```python
from build123d import *

# Parameters (mm, degrees)
SKETCH1_W           = 76.2
SKETCH1_H           = 101.6
SKETCH1_R           = 2.25
BOSS_EXTRUDE1_DEPTH = 3.175
BOSS_EXTRUDE2_DEPTH = 3.175
SKETCH3_R           = 2.25
CUT_EXTRUDE1_DEPTH  = 10


with BuildPart() as part:
    # Sketch1 → Boss-Extrude1 (new body)
    with BuildSketch(Plane(origin=(0, 0, 0), x_dir=(1, 0, 0), z_dir=(0, 1, 0))):
        Rectangle(SKETCH1_W, SKETCH1_H)
        with Locations((-19.05, -41.275)):
            Circle(SKETCH1_R, mode=Mode.SUBTRACT)
        with Locations((19.05, -41.275)):
            Circle(SKETCH1_R, mode=Mode.SUBTRACT)
        with Locations((28.575, -35.56)):
            Circle(SKETCH1_R, mode=Mode.SUBTRACT)
        with Locations((-28.575, -35.56)):
            Circle(SKETCH1_R, mode=Mode.SUBTRACT)
        with Locations((28.575, 35.56)):
            Circle(SKETCH1_R, mode=Mode.SUBTRACT)
        with Locations((19.05, 41.275)):
            Circle(SKETCH1_R, mode=Mode.SUBTRACT)
        with Locations((-28.575, 35.56)):
            Circle(SKETCH1_R, mode=Mode.SUBTRACT)
        with Locations((-19.05, 41.275)):
            Circle(SKETCH1_R, mode=Mode.SUBTRACT)
        with Locations((0, -41.275)):
            Circle(SKETCH1_R, mode=Mode.SUBTRACT)
        with Locations((0, 41.275)):
            Circle(SKETCH1_R, mode=Mode.SUBTRACT)
        with Locations((28.575, 12.7)):
            Circle(SKETCH1_R, mode=Mode.SUBTRACT)
        with Locations((28.575, -12.7)):
            Circle(SKETCH1_R, mode=Mode.SUBTRACT)
        with Locations((22.23, 0)):
            Circle(SKETCH1_R, mode=Mode.SUBTRACT)
    extrude(amount=BOSS_EXTRUDE1_DEPTH)

    # Sketch2 → Boss-Extrude2 (add)
    with BuildSketch(Plane(origin=(0, 3.175, 0), x_dir=(1, 0, 0), z_dir=(0, 1, 0))):
        Polygon((38.1, -50.8), (43.3, -50.8), (43.3, 101.6), (17.9, 101.6), (17.9, 50.8), (38.1, 50.8), align=None)
    extrude(amount=-BOSS_EXTRUDE2_DEPTH)

    # Sketch3 → Cut-Extrude1 (cut)
    with BuildSketch(Plane(origin=(0, 3.175, 0), x_dir=(1, 0, 0), z_dir=(0, 1, 0))):
        with Locations((33.77, 82.55)):
            Circle(SKETCH3_R)
        with Locations((33.77, 69.85)):
            Circle(SKETCH3_R)
        with Locations((27.425, 88.9)):
            Circle(SKETCH3_R)
        with Locations((27.425, 63.5)):
            Circle(SKETCH3_R)
    extrude(amount=-CUT_EXTRUDE1_DEPTH, mode=Mode.SUBTRACT)


solid = part.part
```
Geometry check sheet. Reference: the model listing, model coordinates, mm. A direction names the side the tool comes from. Give positions to 0.01 mm unless a question says otherwise; leave off trailing zeros. Write each loop counter-clockwise with the first axis right and the second up, starting at its lowest first coordinate (ties: lowest second). Pieces come first, ordered by that corner, then holes.
1) Material ranges on L1, parallel to Z at x = 33.77, y = 2.25; L2, parallel to X at y = 1, z = 35.56 (3 decimals); L3, parallel to Z at x = 19.05, y = 1.7 (3 decimals), recorded low to high.
2) Section check A-A, the plane z = -88.9. Record the boundary of the cut face in (x, y) (3 decimals), and give its area (3 significant figures).
3) Section check D-D, the plane x = 28. Record the boundary of the cut face in (y, z) (3 decimals).
4) Access from +Z, -Z, +X, -X, +Y, -Y to the whole of each face (thin tool, end or side, straight path). Record for faces 1 (the flat face through (-10, 2, -50.8)), 2 (the flat face through (-38.1, 2, 1)).
5) Gauge pin test, flat ends, axial feed: pin 1 (5 mm diameter, centred on x = 28.575, z = -35.56, fed in from +Y) (3 decimals); pin 2 (4 mm diameter, centred on x = -19.05, z = 41.275, fed in from -Y); pin 3 (1 mm diameter, centred on y = 1.5, z = -69, fed in from -X); pin 4 (1 mm diameter, centred on x = -9.5, y = 2.5, fed in from -Z). Record the tip position at first contact, or that the pin passes through.
6) Section check C-C, the plane y = 1. State how many separate pieces and enclosed holes the cut face has, and give its area (3 significant figures).
7) Section check B-B, the plane x = 0. Record the boundary of the cut face in (y, z) (3 decimals).
Computed:
1. L1: z = -101.6 to -84.8, -80.3 to -72.1, -67.6 to 50.8
1. L2: x = -38.1 to -30.825, -26.325 to 26.325, 30.825 to 43.3
1. L3: z = -101.6 to -43.525, -39.025 to 39.025, 43.525 to 50.8
2. outline: (17.9, 0) - (25.175, 0) - (25.175, 3.175) - (17.9, 3.175) - close; (29.675, 0) - (43.3, 0) - (43.3, 3.175) - (29.675, 3.175) - close
2. area: 66.4 mm2
3. outline: (0, -101.6) - (3.175, -101.6) - (3.175, -91.075) - (0, -91.075) - close; (0, -86.725) - (3.175, -86.725) - (3.175, -65.675) - (0, -65.675) - close; (0, -61.325) - (3.175, -61.325) - (3.175, -37.735) - (0, -37.735) - close; (0, -33.385) - (3.175, -33.385) - (3.175, -14.875) - (0, -14.875) - close; (0, -10.525) - (3.175, -10.525) - (3.175, 10.525) - (0, 10.525) - close; (0, 14.875) - (3.175, 14.875) - (3.175, 33.385) - (0, 33.385) - close; (0, 37.735) - (3.175, 37.735) - (3.175, 50.8) - (0, 50.8) - close
4. face 1: -Z, -X, +Y, -Y
4. face 2: +Z, -Z, -X, +Y, -Y
5. pin 1: stops at y = 3.175
5. pin 2: passes through
5. pin 3: stops at x = 17.9
5. pin 4: stops at z = -50.8
6. separate pieces: 1
6. enclosed holes: 17
6. area: 9,290 mm2
7. outline: (0, -50.8) - (3.175, -50.8) - (3.175, -43.525) - (0, -43.525) - close; (0, -39.025) - (3.175, -39.025) - (3.175, 39.025) - (0, 39.025) - close; (0, 43.525) - (3.175, 43.525) - (3.175, 50.8) - (0, 50.8) - close
